Model file for the job. Use its own axes, mm. Face numbers are marked on the shaded views. A direction names the side the tool comes from. Coordinates: 2 decimals unless noted, no trailing zeros. Write each loop counter-clockwise with the first axis right and the second up, starting at its lowest first coordinate (ties: lowest second). Pieces come first, ordered by that corner, then holes. Notation, with made-up numbers: (87.25, -9) -> (135.25, -9) arc R14 ccw to (135.25, 6) -> close; hole circle Ø2 at (-24, 16.5). An arc over 180 degrees is marked (long way). Write item = value, one per line. Start each with the question number.
from build123d import *

# Parameters (mm, degrees)
F2_SIZE  = 0.5
F3_R     = 0.5
F6_DEPTH = 4


with BuildPart() as f1:
    # F0 (on Front) → F1 (revolve)
    with BuildSketch(Plane.XZ):
        Polygon((0, 15), (0, 0), (0, -76), (2.5, -78.5), (2.5, -81), (12.5, -81), (12.5, -78.3), (12.5, -77), (12.5, -57), (15, -57), (15, -55.7), (15, -51), (12.5, -51), (12.5, 16), (12.5, 17.1), (12.5, 20), (2.5, 20), (2.5, 17.5), align=None)
    revolve(axis=Axis((0, 0, 55.465363), (0, 0, 1)))

    # F2
    f2_edges = [f1.edges().sort_by_distance(p)[0] for p in [
        (-12.5, 0, 20),
        (-15, 0, -51),
        (-12.5, 0, -51),
        (-12.5, 0, -81),
        (-15, 0, -57),
    ]]
    chamfer(f2_edges, length=F2_SIZE)

    # F3
    f3_edges = [f1.edges().sort_by_distance(p)[0] for p in [
        (-12.5, 0, -57),
    ]]
    fillet(f3_edges, radius=F3_R)

    # F5 (on offset) → F6 (cut)
    with BuildSketch(Plane.XZ.offset(8.5)):
        with BuildLine():
            Line((4, -44.5), (4, 12.5))
            ThreePointArc((4, 12.5), (0, 16.5), (-4, 12.5))
            Line((-4, 12.5), (-4, -44.5))
            ThreePointArc((-4, -44.5), (0, -48.5), (4, -44.5))
        make_face()
    extrude(amount=F6_DEPTH, mode=Mode.SUBTRACT)


solid = f1.part
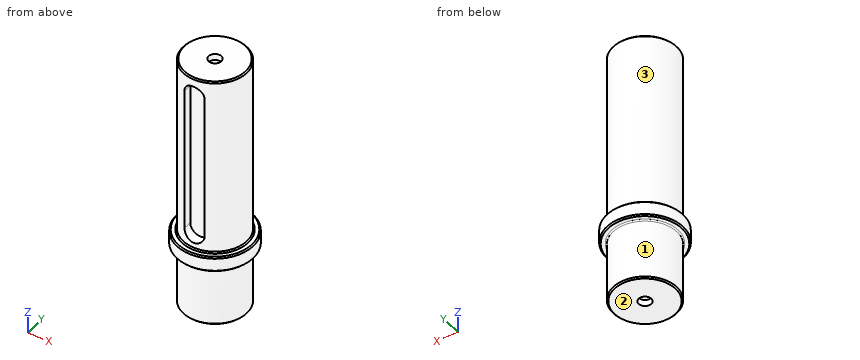
(1) Drop flat-ended pins along their axis: pin 1 Ø8 at (x, z) = (8.5, -20.5) entering from +Y; pin 2 Ø3.5 at (y, z) = (-10, -21.5) entering from -X; pin 3 Ø5 at (y, z) = (7, 4.5) entering from +X; pin 4 Ø1 at (x, y) = (-11.5, -12) entering from +Z. Give the stop position or say it passes through.
(2) Drill centre lines: line 1 along Y through (x, z) = (0, 18.5); line 2 along X through (y, z) = (0.75, -35.5); line 3 along Z through (x, y) = (12, 5.5). Where is each one in solid material? Low to high.
(3) Saw through at C-C (z = -55). Give the cut face in (x, y).
(4) Saw through at B-B (z = -33). Give the cut face in (x, y), then the cut area to 3 significant figures.
(5) Saw through at A-A (z = -73.5). Give the cut face in (x, y), then the cut area to 3 significant figures.
(6) 3-axis set-ups, long thin cutter, end or side, ignore diameter. For the marked faces 1, 2 and 3: which of +Z, -Z, +X, -X, +Y, -Y reach the whole face in a straight line?
Returned:
q1.pin_1 = 11.66
q1.pin_2 = -9.39
q1.pin_3 = 11.66
q1.pin_4 = through
q2.line_1 = -12.5 to -2.5, 2.5 to 12.5
q2.line_2 = -12.48 to 12.48
q2.line_3 = -57 to -51
q3.outline = circle Ø30 at (0, 0)
q4.outline = (-4, -11.84) -> (-4, -8.5) -> (4, -8.5) -> (4, -11.84) arc R12.5 ccw (long way) to start
q4.area = 461 mm2
q5.outline = circle Ø25 at (0, 0)
q5.area = 491 mm2
q6.face_1 = -Z
q6.face_2 = -Z, +X, -X, +Y, -Y
q6.face_3 = +Z
